from build123d import *

# Parameters (mm, degrees)
SKETCH1_R           = 2.5
BOSS_EXTRUDE1_DEPTH = 20
SKETCH1_3_R         = 3.5
BOSS_EXTRUDE2_DEPTH = 2
CHAMFER1_SIZE       = 1
FILLET1_R           = 0.5


with BuildPart() as part:
    # Sketch1 → Boss-Extrude1 (new body)
    with BuildSketch(Plane(origin=(0, 0, 0), x_dir=(0, 1, 0), z_dir=(0, 0, 1))):
        with Locations(Location((0, 0, 0), (0, 0, 270))):
            Circle(SKETCH1_R)
    extrude(amount=-BOSS_EXTRUDE1_DEPTH)

    # Sketch1<3> → Boss-Extrude2 (add)
    with BuildSketch(Plane(origin=(0, 0, 0), x_dir=(0, 1, 0), z_dir=(0, 0, 1))):
        with Locations(Location((0, 0, 0), (0, 0, 270))):
            Circle(SKETCH1_3_R)
    extrude(amount=BOSS_EXTRUDE2_DEPTH)

    # Chamfer1
    chamfer1_edges = [part.edges().sort_by_distance(p)[0] for p in [
        (-3.5, 0, 0),
    ]]
    chamfer(chamfer1_edges, length=CHAMFER1_SIZE - 0.0001)  # a hair under: the kernel refuses the full size

    # Fillet1
    fillet1_edges = [part.edges().sort_by_distance(p)[0] for p in [
        (-3.5, 0, 2),
    ]]
    fillet(fillet1_edges, radius=FILLET1_R)


solid = part.part
Design review of the part built by this model. Coordinates are the model's own, in mm. A direction names the side the tool comes from. Coordinates: 2 decimals unless noted, no trailing zeros. Order: outer loops, then holes, each group sorted by start corner. A loop starts at its lowest first (then second) coordinate and runs counter-clockwise, first axis right, second up.
Item 1: For pin 1 Ø1.5 at (x, z) = (0, -12.5) entering from -Y; pin 2 Ø3 at (y, z) = (0, -13.5) entering from -X; pin 3 Ø2 at (y, z) = (2.5, -10.5) entering from +X, all flat-tipped, find the tip position at first contact; note any pin that passes through.
Item 2: Take a section at C-C, the plane z = -16.25. Write out the cut boundary in (x, y), then the cut area to 3 significant figures.
Item 3: For line 1 (Y direction, x = 0, z = -7); line 2 (Y direction, x = -1.25, z = -12); line 3 (Z direction, x = -2.75, y = -2), list the stretches that pass through material, from the lowest coordinate up.
Item 4: For faces 1 (the flat face through (0, 0, -20)), 2 (the cylindrical face through (-0.54, -2.44, -9.86)), list the 3-axis set-ups (+Z, -Z, +X, -X, +Y, -Y) from which the entire face can be reached by the end or side of a thin tool; tool diameter is ignored.
The answers:
1. pin 1: stops at y = -2.5
1. pin 2: stops at x = -2.5
1. pin 3: stops at x = 2
2. outline: circle Ø5 at (0, 0)
2. area: 19.6 mm2
3. line 1: y = -2.5 to 2.5
3. line 2: y = -2.17 to 2.17
3. line 3: z = 0.9 to 1.8
4. face 1: -Z, +X, -X, +Y, -Y
4. face 2: -Z
